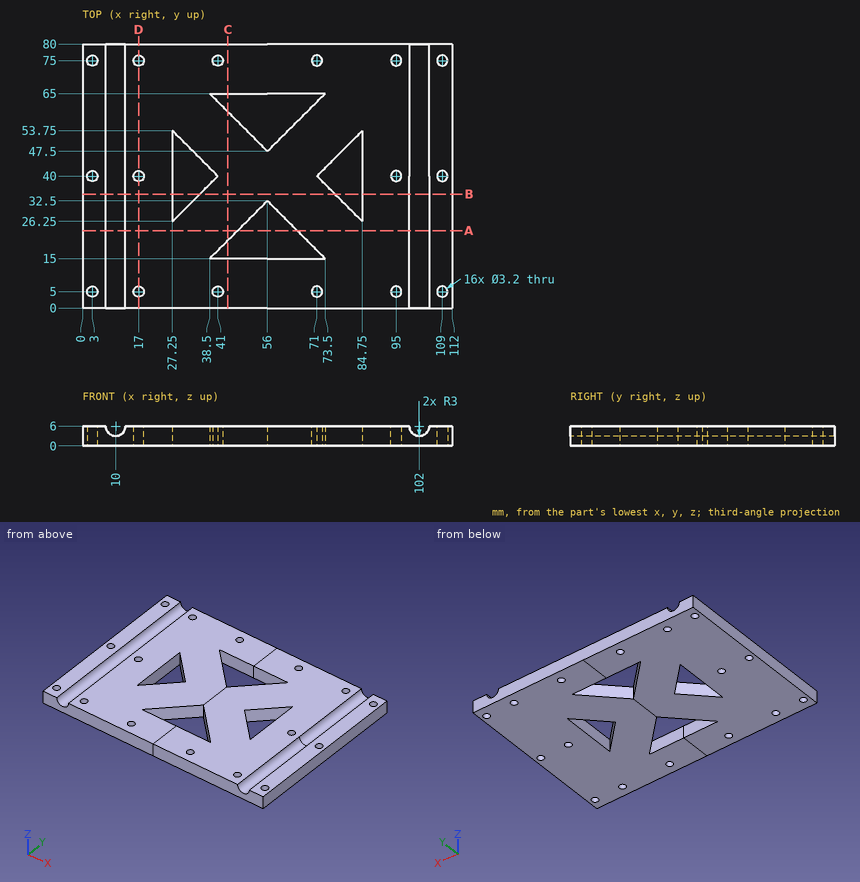
Check sheet for the drawn part. Datum: minimum x, y, z corner. Units: mm. Coordinates: 2 decimals unless noted, no trailing zeros. Write each loop counter-clockwise with the first axis right and the second up, starting at its lowest first coordinate (ties: lowest second). Pieces come first, ordered by that corner, then holes. Notation, with made-up numbers: (52.5, 88.5) - (109.5, 88.5) arc R19 cw to (109.5, 97.5) - close; hole circle Ø1 at (12.25, 32.25). An arc over 180 degrees is marked (long way). Answer as a JSON object with one key per item and string values.
(1) Cross-section at D-D on x = 17. Record the cut outline in (y, z).
Report:
{"outline": "(0, 0) - (3.4, 0) - (3.4, 6) - (0, 6) - close; (6.6, 0) - (38.4, 0) - (38.4, 6) - (6.6, 6) - close; (41.6, 0) - (73.4, 0) - (73.4, 6) - (41.6, 6) - close; (76.6, 0) - (80, 0) - (80, 6) - (76.6, 6) - close"}
(2) Cross-section at A-A on y = 23.5. Record the cut outline in (x, z).
Report:
{"outline": "(0, 0) - (47, 0) - (47, 6) - (13, 6) arc R3 cw to (7, 6) - (0, 6) - close; (65, 0) - (112, 0) - (112, 6) - (105, 6) arc R3 cw to (99, 6) - (65, 6) - close"}
(3) Thickness scan on line 1 along Y through (x, z) = (109, 4.2); line 2 along Y through (x, z) = (33.5, 1.05); line 3 along X through (y, z) = (30, 3.65). Record the ranges inside material, lowest first.
Report:
{"line 1": "0 to 3.4, 6.6 to 38.4, 41.6 to 73.4, 76.6 to 80", "line 2": "0 to 32.5, 47.5 to 80", "line 3": "0 to 8.14, 11.86 to 27.25, 31 to 53.5, 58.5 to 81, 84.75 to 100.14, 103.86 to 112"}
(4) Cross-section at C-C on x = 44. Record the cut outline in (y, z).
Report:
{"outline": "(0, 0) - (15, 0) - (15, 6) - (0, 6) - close; (20.5, 0) - (59.5, 0) - (59.5, 6) - (20.5, 6) - close; (65, 0) - (80, 0) - (80, 6) - (65, 6) - close"}
(5) Cross-section at B-B on y = 34.5. Record the cut outline in (x, z), plus the area to 3 significant figures.
Report:
{"outline": "(0, 0) - (27.25, 0) - (27.25, 6) - (13, 6) arc R3 cw to (7, 6) - (0, 6) - close; (35.5, 0) - (76.5, 0) - (76.5, 6) - (35.5, 6) - close; (84.75, 0) - (112, 0) - (112, 6) - (105, 6) arc R3 cw to (99, 6) - (84.75, 6) - close", "area": "545 mm^2"}
